Can you work these out from the model? Positions are in its coordinate system, mm. Face numbers are marked on the shaded views. A direction names the side the tool comes from. Round coordinates to 2 decimals unless told otherwise and drop trailing zeros. Write each loop counter-clockwise with the first axis right and the second up, starting at its lowest first coordinate (ties: lowest second). Pieces come first, ordered by that corner, then holes. Notation, with made-up numbers: M 74.25,75.5 L 78.25,75.5 A23 ccw 78.25,108.5 Z; hole C 41.5,-10 d2. An arc over 180 degrees is marked long. Answer as a JSON object with one key per item and string values. Group by question number.
1) Suppose I cut it at D-D, the plane x = -8.75. State how many separate pieces and enclosed holes the cut face has, and give its area (3 significant figures).
2) Suppose I cut it at A-A, the plane x = 1.31. Write out the boundary of the cut face in (y, z).
3) Suppose I cut it at B-B, the plane x = 10.25. Write out the boundary of the cut face in (y, z).
4) Please list where these lines run through material, in increasing order: L1, parallel to Y at x = -11, z = 0.3; L2, parallel to Y at x = -1.23, z = 0.3; L3, parallel to Y at x = 8.75, z = 0.2. Write a range as [from, to].
5) Suppose I cut it at C-C, the plane z = 1.3. Write out the boundary of the cut face in (x, y), and give its area (3 significant figures).
6) On a 3-axis mill with a long thin cutter (end or side, diameter ignored), from which of +Z, -Z, +X, -X, +Y, -Y can I reach the whole of each face in a straight line? I mean the marked faces 1 and 2. Say none if no direction works.
7) I'm going to push flat-ended pins straight in: pin 1 Ø1.1 at (x, y) = (3.85, 11.5) entering from -Z; pin 2 Ø3.5 at (x, y) = (4, -12.5) entering from +Z. Where does each tip first touch, or does it pass through?
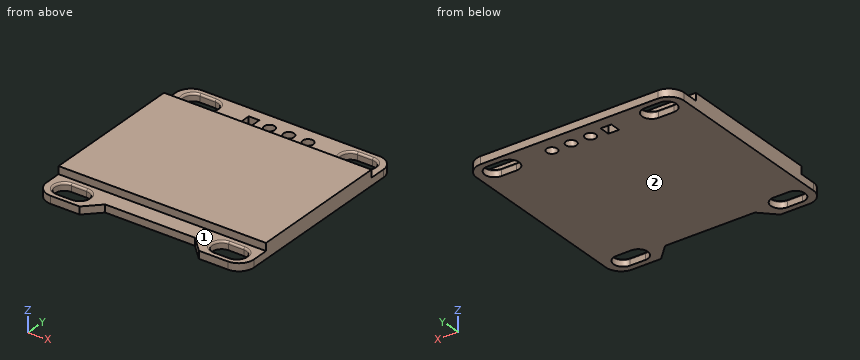
from build123d import *

# Parameters (mm, degrees)
SKETCH1_W           = 27.3
SKETCH1_H           = 27.3
BOSS_EXTRUDE1_DEPTH = 1
FILLET1_R           = 2
CUT_EXTRUDE1_DEPTH  = 2
SKETCH5_W           = 27.3
SKETCH5_H           = 19
BOSS_EXTRUDE2_DEPTH = 1
CUT_EXTRUDE2_DEPTH  = 2
FILLET2_R           = 0.25
SKETCH7_R           = 0.7
SKETCH7_W           = 1.4
SKETCH7_H           = 1.4
CUT_EXTRUDE3_DEPTH  = 1


with BuildPart() as part:
    # Sketch1 → Boss-Extrude1 (new body)
    with BuildSketch(Plane.XY):
        Rectangle(SKETCH1_W, SKETCH1_H)
    extrude(amount=BOSS_EXTRUDE1_DEPTH)

    # Fillet1
    fillet1_edges = [part.edges().sort_by_distance(p)[0] for p in [
        (13.65, -13.65, 0.5),
        (-13.65, -13.65, 0.5),
        (-13.65, 13.65, 0.5),
        (13.65, 13.65, 0.5),
    ]]
    fillet(fillet1_edges, radius=FILLET1_R)

    # Sketch2 → Cut-Extrude1 (cut)
    with BuildSketch(Plane.XY.offset(1)):
        with BuildLine():
            Line((-11.35, 12.85), (-9.35, 12.85))
            ThreePointArc((-9.35, 12.85), (-8.1, 11.6), (-9.35, 10.35))
            Line((-9.35, 10.35), (-11.35, 10.35))
            ThreePointArc((-11.35, 10.35), (-12.6, 11.6), (-11.35, 12.85))
        make_face()
        with BuildLine():
            Line((11.35, 10.35), (9.35, 10.35))
            ThreePointArc((9.35, 10.35), (8.1, 11.6), (9.35, 12.85))
            Line((9.35, 12.85), (11.35, 12.85))
            ThreePointArc((11.35, 12.85), (12.6, 11.6), (11.35, 10.35))
        make_face()
        with BuildLine():
            Line((-11.35, -10.35), (-9.35, -10.35))
            ThreePointArc((-9.35, -10.35), (-8.1, -11.6), (-9.35, -12.85))
            Line((-9.35, -12.85), (-11.35, -12.85))
            ThreePointArc((-11.35, -12.85), (-12.6, -11.6), (-11.35, -10.35))
        make_face()
        with BuildLine():
            Line((11.35, -12.85), (9.35, -12.85))
            ThreePointArc((9.35, -12.85), (8.1, -11.6), (9.35, -10.35))
            Line((9.35, -10.35), (11.35, -10.35))
            ThreePointArc((11.35, -10.35), (12.6, -11.6), (11.35, -12.85))
        make_face()
    extrude(amount=-CUT_EXTRUDE1_DEPTH, mode=Mode.SUBTRACT)

    # Sketch5 → Boss-Extrude2 (add)
    with BuildSketch(Plane.XY.offset(1)):
        Rectangle(SKETCH5_W, SKETCH5_H)
    extrude(amount=BOSS_EXTRUDE2_DEPTH)

    # Sketch3 → Cut-Extrude2 (cut)
    with BuildSketch(Plane.XY.offset(1)):
        Polygon((-7.85, -13.65), (-5.9, -11.7), (5.9, -11.7), (7.85, -13.65), align=None)
    extrude(amount=-CUT_EXTRUDE2_DEPTH, mode=Mode.SUBTRACT)

    # Fillet2
    fillet2_edges = [part.edges().sort_by_distance(p)[0] for p in [
        (12.6, 11.6, 1),
        (10.35, 12.85, 1),
        (8.1, 11.6, 1),
        (10.35, 10.35, 1),
        (-12.6, -11.6, 1),
        (-10.35, -12.85, 1),
        (-8.1, -11.6, 1),
        (-10.35, -10.35, 1),
        (12.6, -11.6, 1),
        (10.35, -10.35, 1),
        (8.1, -11.6, 1),
        (10.35, -12.85, 1),
        (-12.6, 11.6, 1),
        (-10.35, 10.35, 1),
        (-8.1, 11.6, 1),
        (-10.35, 12.85, 1),
    ]]
    fillet(fillet2_edges, radius=FILLET2_R)

    # Sketch7 → Cut-Extrude3 (cut)
    with BuildSketch(Plane(origin=(0, 0, 0), x_dir=(-1, 0, 0), z_dir=(0, 0, -1))):
        with Locations((-3.85, 11.5)):
            Circle(SKETCH7_R)
        with Locations((-1.31, 11.5)):
            Circle(SKETCH7_R)
        with Locations((1.23, 11.5)):
            Circle(SKETCH7_R)
        with Locations((3.77, 11.5)):
            Rectangle(SKETCH7_W, SKETCH7_H)
    extrude(amount=-CUT_EXTRUDE3_DEPTH, mode=Mode.SUBTRACT)


solid = part.part
Results:
{
 "1": {"separate pieces": "3", "enclosed holes": "0", "area": "41.9 mm^2"},
 "2": {"outline": "M -11.7,0 L 10.8,0 L 10.8,1 L 9.5,1 L 9.5,2 L -9.5,2 L -9.5,1 L -11.7,1 Z; M 12.2,0 L 13.65,0 L 13.65,1 L 12.2,1 Z"},
 "3": {"outline": "M -13.65,0 L -12.85,0 L -12.85,0.75 A0.25 ccw -13.1,1 L -13.65,1 Z; M -10.35,0 L 10.35,0 L 10.35,0.75 A0.25 ccw 10.1,1 L 9.5,1 L 9.5,2 L -9.5,2 L -9.5,1 L -10.1,1 A0.25 ccw -10.35,0.75 Z; M 12.85,0 L 13.65,0 L 13.65,1 L 13.1,1 A0.25 ccw 12.85,0.75 Z"},
 "4": {"L1": "[-13.65, -12.85], [-10.35, 10.35], [12.85, 13.65]", "L2": "[-11.7, 10.8], [12.2, 13.65]", "L3": "[-13.65, -12.7], [-10.5, 10.5], [12.7, 13.65]"},
 "5": {"outline": "M -13.65,-9.5 L 13.65,-9.5 L 13.65,9.5 L -13.65,9.5 Z", "area": "519 mm^2"},
 "6": {"face 1": "+Z, +X, -X, -Y", "face 2": "-Z, +X, -X, +Y, -Y"},
 "7": {"pin 1": "through", "pin 2": "z = 1"}
}
